```python
from build123d import *

# Parameters (mm, degrees)
BOSS_EXTRU_1_REACH        = 16.816
BOSS_EXTRU_1_START_RADIUS = 4
BOSS_EXTRU_1_END_RADIUS   = 4
ESQUISSE2_W               = 1.5
ESQUISSE2_H               = 5


with BuildPart() as part:
    # Esquisse1 → Révolution1 (revolve)
    with BuildSketch(Plane.XY):
        Polygon((2.5, 0), (2.5, 10), (0, 10), (0, 11.5), (4, 11.5), (4, 0), align=None)
    revolve(axis=Axis((0, 0, 0), (0, 1, 0)))

    # Boss.-Extru.1: from a cylinder face, 16.816 long prism both ways, kept between that surface and its translate by the depth
    boss_extru_1_start = Plane(origin=(0, 9, 0), z_dir=(0, -1, 0)) * Cylinder(BOSS_EXTRU_1_START_RADIUS, 42.632, mode=Mode.PRIVATE)
    boss_extru_1_end = Plane(origin=(0, 9, 2), z_dir=(0, -1, 0)) * Cylinder(BOSS_EXTRU_1_END_RADIUS, 42.632, mode=Mode.PRIVATE)
    # Esquisse2 → Boss.-Extru.1 (add, from a surface)
    with BuildSketch(Plane.XY, mode=Mode.PRIVATE) as boss_extru_1_sk1:
        with Locations((0, 9)):
            Rectangle(ESQUISSE2_W, ESQUISSE2_H)
    boss_extru_1_tool1 = extrude(boss_extru_1_sk1.sketch, amount=BOSS_EXTRU_1_REACH, both=True, mode=Mode.PRIVATE)
    add(((boss_extru_1_tool1 - boss_extru_1_start) & boss_extru_1_end).solids().sort_by_distance((0, 9, 4.929058))[0])


solid = part.part
```
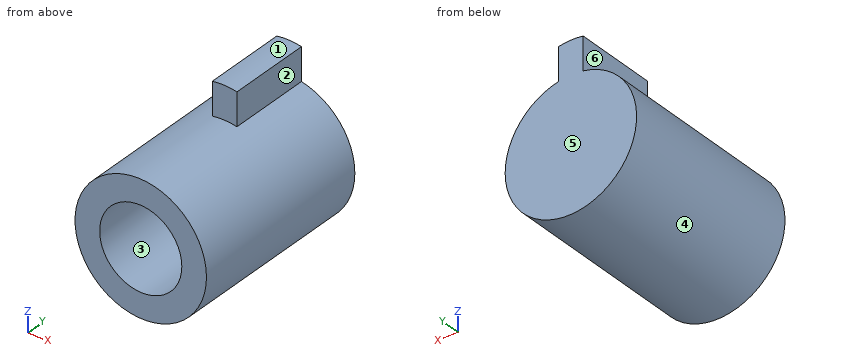
For this review, take the finished solid that the model builds, in its own axes (mm). Face numbers are marked on the shaded views. A direction names the side the tool comes from. Coordinates: 2 decimals unless noted, no trailing zeros. Write each loop counter-clockwise with the first axis right and the second up, starting at its lowest first coordinate (ties: lowest second). Pieces come first, ordered by that corner, then holes.
(1) Add section B-B on y = 7.75. Give the boundary of the cut face in (x, z).
(2) Add section D-D on z = 1.25. Give the boundary of the cut face in (x, y), then the cut area to 3 significant figures.
(3) Add section C-C on x = 0. Give the boundary of the cut face in (y, z), then the cut area to 3 significant figures.
(4) Wall thickness on probe 1 along X at (y, z) = (7, 0); probe 2 along Z at (x, y) = (0, 8); probe 3 along Y at (x, z) = (-0.5, 0): over which ranges is each line inside the solid? List them lowest first.
(5) The part is to be moulded in two halves that separate along Z. For the marked faces 1, 2, 3 and 4, say which applies: +Z half, -Z half, draft (parallel to the pull), parting line (faces both ways), or undercut.
(6) For pin 1 Ø2 at (x, y) = (-1.5, 7) entering from -Z; pin 2 Ø4 at (x, z) = (0.5, -1) entering from -Y; pin 3 Ø0.6 at (y, z) = (9.5, 5) entering from +X; pin 4 Ø0.6 at (y, z) = (10, 5.5) entering from -X, all flat-tipped, find the tip position at first contact; note any pin that passes through.
(7) Tool access review of the marked faces 5 and 6: name each direction out of +Z, -Z, +X, -X, +Y, -Y from which nothing blocks a thin tool from reaching the whole face with its end or side.
(8) Add section A-A on z = 0. Give the boundary of the cut face in (x, y).
Answer sheet:
1. outline: (-0.75, 3.93) arc R4 ccw (long way) to (0.75, 3.93) - (0.75, 5.93) arc R4 ccw to (-0.75, 5.93) - close; hole circle Ø5 at (0, 0)
2. outline: (-3.8, 0) - (-2.17, 0) - (-2.17, 10) - (2.17, 10) - (2.17, 0) - (3.8, 0) - (3.8, 11.5) - (-3.8, 11.5) - close
2. area: 44.1 mm2
3. outline: (0, -4) - (11.5, -4) - (11.5, 6) - (6.5, 6) - (6.5, 4) - (0, 4) - (0, 2.5) - (10, 2.5) - (10, -2.5) - (0, -2.5) - close
3. area: 52.0 mm2
4. probe 1: x = -4 to -2.5, 2.5 to 4
4. probe 2: z = -4 to -2.5, 2.5 to 6
4. probe 3: y = 10 to 11.5
5. face 1: +Z half
5. face 2: draft
5. face 3: undercut
5. face 4: parting line
6. pin 1: stops at z = -3.97
6. pin 2: stops at y = 0
6. pin 3: stops at x = 0.75
6. pin 4: stops at x = -0.75
7. face 5: +Z, -Z, +X, -X, +Y
7. face 6: +Z, -X, +Y, -Y
8. outline: (-4, 0) - (-2.5, 0) - (-2.5, 10) - (2.5, 10) - (2.5, 0) - (4, 0) - (4, 11.5) - (-4, 11.5) - close
